Design review of the part built by this model. Coordinates are the model's own, in mm. A direction names the side the tool comes from. Give positions to 0.01 mm unless a question says otherwise; leave off trailing zeros. Loops run counter-clockwise (first coordinate to the right, second up) from the corner with the lowest first, then second, coordinate; pieces in that order, holes last. Notation, with made-up numbers: M 67.25,84 L 76.25,84 A3 cw 76.25,88 Z; hole C 38,81.5 d6. An arc over 180 degrees is marked long. Use a Markdown table: item, result. Add a question column.
(1) Draft analysis for pull direction X (two halves, no side actions). For faces 1 (the face through (-16.115, 14.132, 0.986)), 2 (the face through (-43.03, 28.21, 0.99)), state which applies: pulls with the +X half, pulls with the -X half, needs draft (parallel to the pull), parting line crosses it, or undercut.
(2) Add section C-C, the plane y = 19. Give the boundary of the cut face in (x, z), then the cut area to 3 significant figures.
(3) Add section D-D, the plane z = 0.35. State how many separate pieces and enclosed holes the cut face has, then the cut area to 3 significant figures.
(4) Add section B-B, the plane x = -42. Give the boundary of the cut face in (y, z), then the cut area to 3 significant figures.
(5) For faces 3 (the face through (-32.92, 28.665, 0.986)), 4 (the face through (42, -0.09, 1)), 5 (the face through (0.366, 6.255, 0.986)), list the 3-axis set-ups (+Z, -Z, +X, -X, +Y, -Y) from which the entire face can be reached by the end or side of a thin tool; tool diameter is ignored.
(6) Add section A-A, the plane y = 28. Give the boundary of the cut face in (x, z).
(7) For probe 1 along X at (y, z) = (2, 1.4); probe 2 along X at (y, z) = (15.5, 1.4); probe 3 along Y at (x, z) = (41, 1.95), list the stretches that pass through material, from the lowest coordinate up.
```python
from build123d import *

# Parameters (mm, degrees)
SKETCH_3_R      = 2.2
SKETCH_3_R_2    = 1.5
EXTRUDE_1_DEPTH = 2


with BuildPart() as part:
    # 草图3 → 凸台-拉伸1 (new body)
    with BuildSketch(Plane.XY):
        with BuildLine():
            Line((-41, -4.490216685), (-42, -4.490216685))
            Line((-42, -4.490216685), (-44, -4.490216685))
            Line((-44, -4.490216685), (-45, -4.490216685))
            Line((-45, -4.490216685), (-45, 4.509783315))
            Line((-45, 4.509783315), (-45, 14.509783315))
            Line((-45, 14.509783315), (-45, 26.463053661))
            Line((-45, 26.463053661), (-41, 30.009783315))
            ThreePointArc((-41, 30.009783315), (-32.811469568, 28.6216516), (-25.896750373, 24.021043081))
            ThreePointArc((-25.896750373, 24.021043081), (-15.928379069, 14.053074936), (-1.831258252, 14.053360012))
            ThreePointArc((-1.831258252, 14.053360012), (0, 14.009783315), (1.831258252, 14.053360012))
            ThreePointArc((1.831258252, 14.053360012), (15.928379069, 14.053074936), (25.896750373, 24.021043081))
            ThreePointArc((25.896750373, 24.021043081), (32.811469568, 28.6216516), (41, 30.009783315))
            Line((41, 30.009783315), (45, 26.463053661))
            Line((45, 26.463053661), (45, 14.509783315))
            Line((45, 14.509783315), (45, 4.509783315))
            Line((45, 4.509783315), (45, -4.490216685))
            Line((45, -4.490216685), (41, -4.490216685))
            Line((41, -4.490216685), (25.7, -4.490216685))
            Line((25.7, -4.490216685), (25.7, -0.390216685))
            Line((25.7, -0.390216685), (25.7, 2.109783315))
            ThreePointArc((25.7, 2.109783315), (0, 6.256082772), (-25.7, 2.109783315))
            Line((-25.7, 2.109783315), (-25.7, -0.390216685))
            Line((-25.7, -0.390216685), (-25.7, -4.490216685))
            Line((-25.7, -4.490216685), (-41, -4.490216685))
        make_face()
        with Locations((0, 10.509783315)):
            Circle(SKETCH_3_R, mode=Mode.SUBTRACT)
        with Locations((-29.69848481, 22.811298505)):
            Circle(SKETCH_3_R, mode=Mode.SUBTRACT)
        with Locations((-26.8, 9.509783315)):
            Circle(SKETCH_3_R_2, mode=Mode.SUBTRACT)
        with Locations(Location((26.8, 9.509783315, 0), (0, 0, 180))):
            Circle(SKETCH_3_R_2, mode=Mode.SUBTRACT)
        with Locations((-42, 10.009783315)):
            Circle(SKETCH_3_R_2, mode=Mode.SUBTRACT)
        with Locations(Location((42, 10.009783315, 0), (0, 0, 180))):
            Circle(SKETCH_3_R_2, mode=Mode.SUBTRACT)
        with Locations((29.69848481, 22.811298505)):
            Circle(SKETCH_3_R, mode=Mode.SUBTRACT)
        with BuildLine():
            Line((-37.1, -2.090216685), (-29.9, -2.090216685))
            Line((-29.9, -2.090216685), (-29.9, 0.109783315))
            Line((-29.9, 0.109783315), (-37.1, 0.109783315))
            ThreePointArc((-37.1, 0.109783315), (-37.555634919, -0.990216685), (-37.1, -2.090216685))
        make_face(mode=Mode.SUBTRACT)
        with BuildLine():
            Line((29.9, -2.090216685), (29.9, 0.109783315))
            Line((29.9, 0.109783315), (37.1, 0.109783315))
            ThreePointArc((37.1, 0.109783315), (37.555634919, -0.990216685), (37.1, -2.090216685))
            Line((37.1, -2.090216685), (29.9, -2.090216685))
        make_face(mode=Mode.SUBTRACT)
        with BuildLine():
            Line((-43.1, 5.109783315), (-43.1, -0.090216685))
            Line((-43.1, -0.090216685), (-40.9, -0.090216685))
            Line((-40.9, -0.090216685), (-40.9, 5.109783315))
            ThreePointArc((-40.9, 5.109783315), (-42, 5.565418233), (-43.1, 5.109783315))
        make_face(mode=Mode.SUBTRACT)
        with BuildLine():
            Line((-43.1, 20.109783315), (-40.9, 20.109783315))
            Line((-40.9, 20.109783315), (-40.9, 14.909783315))
            ThreePointArc((-40.9, 14.909783315), (-42, 14.454148396), (-43.1, 14.909783315))
            Line((-43.1, 14.909783315), (-43.1, 20.109783315))
        make_face(mode=Mode.SUBTRACT)
        with BuildLine():
            Line((40.9, 20.109783315), (40.9, 14.909783315))
            ThreePointArc((40.9, 14.909783315), (42, 14.454148396), (43.1, 14.909783315))
            Line((43.1, 14.909783315), (43.1, 20.109783315))
            Line((43.1, 20.109783315), (40.9, 20.109783315))
        make_face(mode=Mode.SUBTRACT)
        with BuildLine():
            Line((40.9, 5.109783315), (40.9, -0.090216685))
            Line((40.9, -0.090216685), (43.1, -0.090216685))
            Line((43.1, -0.090216685), (43.1, 5.109783315))
            ThreePointArc((43.1, 5.109783315), (42, 5.565418233), (40.9, 5.109783315))
        make_face(mode=Mode.SUBTRACT)
    extrude(amount=EXTRUDE_1_DEPTH)


solid = part.part
```
Established:
| question | item | result |
|---|---|---|
| 1 | face 1 | undercut |
| 1 | face 2 | pulls with the -X half |
| 2 | outline | M -45,0 L -43.1,0 L -43.1,2 L -45,2 Z; M -40.9,0 L -22.79,0 L -22.79,2 L -40.9,2 Z; M 22.79,0 L 40.9,0 L 40.9,2 L 22.79,2 Z; M 43.1,0 L 45,0 L 45,2 L 43.1,2 Z |
| 2 | area | 80.0 mm^2 |
| 3 | separate pieces | 1 |
| 3 | enclosed holes | 13 |
| 3 | area | 1,620 mm^2 |
| 4 | outline | M -4.49,0 L -0.09,0 L -0.09,2 L -4.49,2 Z; M 5.57,0 L 8.51,0 L 8.51,2 L 5.57,2 Z; M 11.51,0 L 14.45,0 L 14.45,2 L 11.51,2 Z; M 20.11,0 L 29.12,0 L 29.12,2 L 20.11,2 Z |
| 4 | area | 38.6 mm^2 |
| 5 | face 3 | +Z, -Z, +Y |
| 5 | face 4 | +Z, -Z |
| 5 | face 5 | +Z, -Z, -Y |
| 6 | outline | M -43.27,0 L -31.4,0 L -31.4,2 L -43.27,2 Z; M 31.4,0 L 43.27,0 L 43.27,2 L 31.4,2 Z |
| 7 | probe 1 | -45 to -43.1, -40.9 to -25.7, 25.7 to 40.9, 43.1 to 45 |
| 7 | probe 2 | -45 to -43.1, -40.9 to -18.72, 18.72 to 40.9, 43.1 to 45 |
| 7 | probe 3 | -4.49 to -0.09, 5.2 to 8.89, 11.13 to 14.82, 20.11 to 30.01 |
